Source: CAD feature listing. Evaluate the final solid. Frame: model axes, mm. A direction names the side the tool comes from. Coordinates: 2 decimals unless noted, no trailing zeros. Order: outer loops, then holes, each group sorted by start corner. A loop starts at its lowest first (then second) coordinate and runs counter-clockwise, first axis right, second up. Notation, with made-up numbers: (62.25, -33) -> (121.25, -33) arc R30 ccw to (121.25, -2) -> close; hole circle Ø5 at (-11, 0.25). An arc over 180 degrees is marked (long way). Put each result on its own line as item: value.
from build123d import *

# Parameters (mm, degrees)
CROQUIS3_R                                           = 3
SALIENTE_EXTRUIR1_DEPTH                              = 5
CROQUIS3_R_2                                         = 2.5
SALIENTE_EXTRUIR1_2_DEPTH                            = 5
SALIENTE_EXTRUIR1_3_DEPTH                            = 5
TALADRO_DE_MARGEN_PARA_M21_AT_2_COUNT                = 2
TALADRO_DE_MARGEN_PARA_M21_AT_2_PITCH                = 83.855175288
TALADRO_DE_MARGEN_PARA_M21_AT_3_COUNT                = 2
TALADRO_DE_MARGEN_PARA_M21_AT_3_PITCH                = 80.670217057
CROQUIS9_R                                           = 1.8
CROQUIS9_R_2                                         = 1.225
SALIENTE_EXTRUIR3_DEPTH                              = 1
SALIENTE_EXTRUIR4_DEPTH                              = 4
SALIENTE_EXTRUIR5_DEPTH                              = 30
SALIENTE_EXTRUIR5_DEPTH_BACK                         = 4
CORTAR_EXTRUIR2_DEPTH                                = 5
CROQUIS13_R                                          = 10
CORTAR_EXTRUIR3_DEPTH                                = 5
REDONDEO1_R                                          = 4
SALIENTE_EXTRUIR9_START                              = 30
CROQUIS15_R                                          = 4
SALIENTE_EXTRUIR9_DEPTH                              = 30
REFRENTADO_PARA_TORNILLO_TAP_N_CON_CABEZ_D           = 2.5
REFRENTADO_PARA_TORNILLO_TAP_N_CON_CABEZ_DEPTH       = 10
REFRENTADO_PARA_TORNILLO_TAP_N_CON_CABEZ_CSINK_D     = 4
REFRENTADO_PARA_TORNILLO_TAP_N_CON_CABEZ_CSINK_ANGLE = 90
REFRENTADO_PARA_TORNILLO_TAP_N_CON_CABEZ_TIP         = 0.751075774
REFRENTADO_PARA_TORNILLO_TAP_N_CON_C_2_D             = 4.5
REFRENTADO_PARA_TORNILLO_TAP_N_CON_C_2_DEPTH         = 10
REFRENTADO_PARA_TORNILLO_TAP_N_CON_C_2_CSINK_D       = 8.96
REFRENTADO_PARA_TORNILLO_TAP_N_CON_C_2_CSINK_ANGLE   = 90
REFRENTADO_PARA_TORNILLO_TAP_N_CON_C_2_TIP           = 1.351936393


with BuildPart() as part:
    # Croquis3 → Saliente-Extruir1 (new body)
    with BuildSketch(Plane(origin=(0, 0, 0), x_dir=(1, 0, 0), z_dir=(0, 1, 0))):
        with Locations(Location((5.2388, 19.05, 0), (0, 0, 270))):
            Circle(CROQUIS3_R)
    extrude(amount=SALIENTE_EXTRUIR1_DEPTH)

    # Croquis8 → Taladro de margen para M21 (revolve, cut)
    with BuildSketch(Plane(origin=(5.2388, 5, -19.05), x_dir=(0, 0, 1), z_dir=(1, 0, 0))):
        Polygon((0, 0), (0, 5), (1.2, 5), (1.2, 0.025), (1.225, 0), align=None)
    taladro_de_margen_para_m21 = revolve(axis=Axis((5.2388, 11.35, -19.05), (0, -1, 0)), mode=Mode.SUBTRACT)

    # Croquis9 → Saliente-Extruir3 (add)
    with BuildSketch(Plane(origin=(0, 5, 0), x_dir=(1, 0, 0), z_dir=(0, 1, 0))):
        with Locations(Location((5.2388, 19.05, 0), (0, 0, 270))):
            Circle(CROQUIS9_R)
        with Locations(Location((5.2388, 19.05, 0), (0, 0, 270))):
            Circle(CROQUIS9_R_2, mode=Mode.SUBTRACT)
    extrude(amount=SALIENTE_EXTRUIR3_DEPTH)



with BuildPart() as body_2:
    # Croquis3 → Saliente-Extruir1 2 (new body)
    with BuildSketch(Plane(origin=(0, 0, 0), x_dir=(1, 0, 0), z_dir=(0, 1, 0))):
        with Locations(Location((85.2488, 44.1516, 0), (0, 0, 270))):
            Circle(CROQUIS3_R_2)
    extrude(amount=SALIENTE_EXTRUIR1_2_DEPTH)

    # Taladro de margen para M21 at 2: Taladro de margen para M21 ×2
    with Locations(*[Vector(0.9541450450175183, 0, -0.2993446726910604) * (i * TALADRO_DE_MARGEN_PARA_M21_AT_2_PITCH) for i in range(1, TALADRO_DE_MARGEN_PARA_M21_AT_2_COUNT)]):
        add(taladro_de_margen_para_m21, mode=Mode.SUBTRACT)


with BuildPart() as body_3:
    # Croquis3 → Saliente-Extruir1 3 (new body)
    with BuildSketch(Plane(origin=(0, 0, 0), x_dir=(1, 0, 0), z_dir=(0, 1, 0))):
        with Locations(Location((85.2488, 8.7503, 0), (0, 0, 270))):
            Circle(CROQUIS3_R_2)
    extrude(amount=SALIENTE_EXTRUIR1_3_DEPTH)

    # Taladro de margen para M21 at 3: Taladro de margen para M21 ×2
    with Locations(*[Vector(0.9918158512336425, 0, 0.12767661196039432) * (i * TALADRO_DE_MARGEN_PARA_M21_AT_3_PITCH) for i in range(1, TALADRO_DE_MARGEN_PARA_M21_AT_3_COUNT)]):
        add(taladro_de_margen_para_m21, mode=Mode.SUBTRACT)


with BuildPart() as part_1:
    add(part.part)

    add(body_2.part)  # Saliente-Extruir4 merges body 2

    add(body_3.part)  # Saliente-Extruir4 merges body 3
    # Croquis10 → Saliente-Extruir4 (add)
    with BuildSketch(Plane(origin=(0, 0, 0), x_dir=(1, 0, 0), z_dir=(0, 1, 0))):
        Polygon((-10, -10), (100.17, -10), (100.17, 62.7203), (-54.8412, 62.7203), (-54.8412, 30), (-10, 30), align=None)
    extrude(amount=-SALIENTE_EXTRUIR4_DEPTH)

    # Croquis11 → Saliente-Extruir5 (add, two sides: drawn at the far end of the back side and taken through both)
    with BuildSketch(Plane(origin=(0, 0, 0), x_dir=(1, 0, 0), z_dir=(0, 1, 0)).offset(-SALIENTE_EXTRUIR5_DEPTH_BACK)):
        Polygon((104.17, -14), (104.17, 66.7203), (-58.8412, 66.7203), (-58.8412, 26), (-58.8412, 22), (-14, 22), (-14, -14), align=None)
        Polygon((100.17, -10), (100.17, 62.7203), (-54.8412, 62.7203), (-54.8412, 30), (-10, 30), (-10, -10), align=None, mode=Mode.SUBTRACT)
    extrude(amount=SALIENTE_EXTRUIR5_DEPTH + SALIENTE_EXTRUIR5_DEPTH_BACK)

    # Croquis12 → Cortar-Extruir2 (cut)
    with BuildSketch(Plane.XY.offset(-22)):
        Polygon((-21.430218943, 15), (-27.925409472, 26.25), (-40.915790528, 26.25), (-47.410981057, 15), (-40.915790528, 3.75), (-27.925409472, 3.75), align=None)
    extrude(amount=-CORTAR_EXTRUIR2_DEPTH, mode=Mode.SUBTRACT)

    # Croquis13 → Cortar-Extruir3 (cut)
    with BuildSketch(Plane.XY.offset(-27)):
        with Locations((-34.4206, 15)):
            Circle(CROQUIS13_R)
    extrude(amount=-CORTAR_EXTRUIR3_DEPTH, mode=Mode.SUBTRACT)

    # Redondeo1
    redondeo1_edges = [part_1.edges().sort_by_distance(p)[0] for p in [
        (-54.8412, 15, -62.7203),
        (-54.8412, 15, -30),
        (-10, 15, -30),
        (100.17, 15, 10),
        (-10, 15, 10),
        (100.17, 15, -62.7203),
        (104.17, 13, 14),
        (45.085, -4, 14),
        (-14, 13, 14),
        (-14, -4, -4),
        (-36.4206, -4, -22),
        (-58.8412, 13, -22),
        (-58.8412, -4, -44.36015),
        (-58.8412, 13, -66.7203),
        (22.6644, -4, -66.7203),
        (104.17, 13, -66.7203),
        (104.17, -4, -26.36015),
    ]]
    fillet(redondeo1_edges, radius=REDONDEO1_R)

    # Croquis15 → Saliente-Extruir9 (add)
    with BuildSketch(Plane(origin=(0, 0, 0), x_dir=(1, 0, 0), z_dir=(0, 1, 0)).offset(SALIENTE_EXTRUIR9_START)):
        with Locations((-54.8412, 62.7203)):
            Circle(CROQUIS15_R)
        with Locations((100.17, 62.7203)):
            Circle(CROQUIS15_R)
        with Locations((100.17, -10)):
            Circle(CROQUIS15_R)
        with Locations((-10, -10)):
            Circle(CROQUIS15_R)
        with Locations((-14, 26)):
            Circle(CROQUIS15_R)
        with Locations((-54.8412, 26)):
            Circle(CROQUIS15_R)
        with Locations((22.6644, 62.7203)):
            Circle(CROQUIS15_R)
    extrude(amount=-SALIENTE_EXTRUIR9_DEPTH)

    # Refrentado para tornillo tap_n con cabez
    with Locations(Plane(origin=(0, 30, 0), x_dir=(1, 0, 0), z_dir=(0, 1, 0))):
        with Locations((-54.8412, 62.7203), (-54.8412, 26), (-14, 26), (-10, -10), (100.17, -10), (100.17, 62.7203), (22.6644, 62.7203)):
            CounterSinkHole(REFRENTADO_PARA_TORNILLO_TAP_N_CON_CABEZ_D / 2, REFRENTADO_PARA_TORNILLO_TAP_N_CON_CABEZ_CSINK_D / 2, depth=REFRENTADO_PARA_TORNILLO_TAP_N_CON_CABEZ_DEPTH, counter_sink_angle=REFRENTADO_PARA_TORNILLO_TAP_N_CON_CABEZ_CSINK_ANGLE)
            with Locations((0, 0, -(REFRENTADO_PARA_TORNILLO_TAP_N_CON_CABEZ_DEPTH + REFRENTADO_PARA_TORNILLO_TAP_N_CON_CABEZ_TIP / 2))):  # 118° drill point
                Cone(0, REFRENTADO_PARA_TORNILLO_TAP_N_CON_CABEZ_D / 2, REFRENTADO_PARA_TORNILLO_TAP_N_CON_CABEZ_TIP, mode=Mode.SUBTRACT)

    # Refrentado para tornillo tap_n con c 2
    with Locations(Plane(origin=(0, 0, 0), x_dir=(1, 0, 0), z_dir=(0, 1, 0))):
        with Locations((5, 54.7203), (85.17, 54.7203), (85.17, -2), (5, -2)):
            CounterSinkHole(REFRENTADO_PARA_TORNILLO_TAP_N_CON_C_2_D / 2, REFRENTADO_PARA_TORNILLO_TAP_N_CON_C_2_CSINK_D / 2, depth=REFRENTADO_PARA_TORNILLO_TAP_N_CON_C_2_DEPTH, counter_sink_angle=REFRENTADO_PARA_TORNILLO_TAP_N_CON_C_2_CSINK_ANGLE)
            with Locations((0, 0, -(REFRENTADO_PARA_TORNILLO_TAP_N_CON_C_2_DEPTH + REFRENTADO_PARA_TORNILLO_TAP_N_CON_C_2_TIP / 2))):  # 118° drill point
                Cone(0, REFRENTADO_PARA_TORNILLO_TAP_N_CON_C_2_D / 2, REFRENTADO_PARA_TORNILLO_TAP_N_CON_C_2_TIP, mode=Mode.SUBTRACT)


solid = part_1.part
1. Cut plane B-B on x = 55. Output: boundary loops of the cut face in (y, z), plus the area to 3 significant figures.
Numbers:
outline: (-4, -62.72) arc R4 ccw to (0, -66.72) -> (30, -66.72) -> (30, -62.72) -> (0, -62.72) -> (0, 10) -> (30, 10) -> (30, 14) -> (0, 14) arc R4 ccw to (-4, 10) -> close
area: 556 mm2
2. Set-up query: faces 5 (the cylindrical face through (-57.7, 15.2, -23.2)), 6 (the flat face through (-24.72, 9.3, -24.46)), 7 (the cylindrical face through (6.14, 2.46, -16.19)). Return all of +Z, -Z, +X, -X, +Y, -Y with unobstructed straight access to the full face (end or side cutting, diameter ignored); none if empty.
Numbers:
face 5: +Z, -X, +Y, -Y
face 6: +Z
face 7: +Y
3. Pull-direction query (Y, two-part tool) for faces 1 (the flat face through (-24.632, 20.546, -24.465)), 2 (the flat face through (-44.12, 20.7, -24.46)), 3 (the flat face through (-44, 8, -22)), 4 (the conical face through (82.92, -2.12, -55.43)); classes: pulls with the +Y half, pulls with the -Y half, needs draft (parallel to the pull), parting line crosses it, or undercut.
Numbers:
face 1: undercut
face 2: undercut
face 3: needs draft
face 4: pulls with the +Y half
4. Ray query, line 1 along X through (y, z) = (2, -19); line 2 along Z through (x, y) = (79.5, 15.5); line 3 along Z through (x, y) = (100, 26). Return the intervals inside material, ascending.
Numbers:
line 1: x = -14 to -10, 2.24 to 4.04, 6.44 to 8.24, 100.17 to 104.17
line 2: z = -66.72 to -62.72, 10 to 14
line 3: z = -66.72 to -63.96, -61.48 to -58.72, 6 to 8.76, 11.24 to 14
5. Cut plane A-A on z = 2. Output: boundary loops of the cut face in (x, y), plus the area to 3 significant figures.
Numbers:
outline: (-14, 0) arc R4 ccw to (-10, -4) -> (2.75, -4) -> (2.75, -2.23) -> (0.52, 0) -> (-10, 0) -> (-10, 30) -> (-14, 30) -> close; (7.25, -4) -> (82.92, -4) -> (82.92, -2.23) -> (80.69, 0) -> (9.48, 0) -> (7.25, -2.23) -> close; (87.42, -4) -> (100.17, -4) arc R4 ccw to (104.17, 0) -> (104.17, 30) -> (100.17, 30) -> (100.17, 0) -> (89.65, 0) -> (87.42, -2.23) -> close
area: 660 mm2
6. First-contact query: pin 1 (12 mm diameter, centred on x = -26.5, z = -48, fed in from +Y); pin 2 (5 mm diameter, centred on x = 5, z = -54.72, fed in from +Y); pin 3 (4 mm diameter, centred on x = 86, z = -44, fed in from +Y). Flat tips, straight axial feed; report the tip coordinate or a pass-through.
Numbers:
pin 1: stops at y = 0
pin 2: stops at y = -1.98
pin 3: stops at y = 5
